Read the model definition and answer for the solid it produces. Units are mm, in the model's axes. Face numbers are marked on the shaded views. A direction names the side the tool comes from. Coordinates: 2 decimals unless noted, no trailing zeros. Write each loop counter-clockwise with the first axis right and the second up, starting at its lowest first coordinate (ties: lowest second). Pieces come first, ordered by that corner, then holes. Notation, with made-up numbers: (61, 71.25) -> (113, 71.25) arc R21 ccw to (113, 89.25) -> close; hole circle Ø1 at (66, 41). An arc over 180 degrees is marked (long way). One line per item, written item: value. Start each with the question number.
from build123d import *

# Parameters (mm, degrees)
SALIENTE_EXTRUIR1_DEPTH = 18
CROQUIS2_R              = 2.5
CORTAR_EXTRUIR1_DEPTH   = 2.5
CROQUIS3_W              = 13
CROQUIS3_H              = 3
CORTAR_EXTRUIR2_DEPTH   = 47.14108798
CHAFL_N1_SIZE           = 1
CHAFL_N2_SIZE           = 1
CHAFL_N2_SIZE2          = 2.087588248
CROQUIS4_W              = 8
CROQUIS4_H              = 12
SALIENTE_EXTRUIR2_DEPTH = 2
CROQUIS5_R              = 1
CORTAR_EXTRUIR3_DEPTH   = 46.169126624
CHAFL_N3_SIZE           = 3
CHAFL_N4_SIZE           = 2


with BuildPart() as part:
    # Croquis1 → Saliente-Extruir1 (new body)
    with BuildSketch(Plane(origin=(0, 0, 0), x_dir=(1, 0, 0), z_dir=(0, 1, 0))):
        Polygon((4, -1.5), (38, -17.5), (38, -14.5), (4, 1.5), (-4, 1.5), (-4, -1.5), align=None)
    extrude(amount=SALIENTE_EXTRUIR1_DEPTH)

    # Croquis2 → Cortar-Extruir1 (cut)
    with BuildSketch(Plane(origin=(0, 0, -1.5), x_dir=(-1, 0, 0), z_dir=(0, 0, -1))):
        with Locations((0, 9)):
            Circle(CROQUIS2_R)
    extrude(amount=-CORTAR_EXTRUIR1_DEPTH, mode=Mode.SUBTRACT)

    # Croquis3 → Cortar-Extruir2 (cut, through all)
    with BuildSketch(Plane(origin=(0, 0, -1.5), x_dir=(-1, 0, 0), z_dir=(0, 0, -1))):
        with Locations((-2.5, 16.5)):
            Rectangle(CROQUIS3_W, CROQUIS3_H)
        with Locations((-2.5, 1.5)):
            Rectangle(CROQUIS3_W, CROQUIS3_H)
    extrude(amount=-CORTAR_EXTRUIR2_DEPTH, mode=Mode.SUBTRACT)

    # Chaflán1
    chafl_n1_edges = [part.edges().sort_by_distance(p)[0] for p in [
        (23.5, 18, 7.676470588),
        (23.5, 0, 7.676470588),
    ]]
    chamfer(chafl_n1_edges, length=CHAFL_N1_SIZE)

    # Chaflán2
    chafl_n2_edges = [part.edges().sort_by_distance(p)[0] for p in [
        (38, 9, 14.5),
    ]]
    chafl_n2_side = [part.faces().sort_by_distance(p)[0] for p in [
        (38, 9, 16.023643901),
    ]]
    chamfer(chafl_n2_edges, length=CHAFL_N2_SIZE, length2=CHAFL_N2_SIZE2, reference=chafl_n2_side[0])

    # Croquis4 → Saliente-Extruir2 (add)
    with BuildSketch(Plane.XY.offset(1.5)):
        with Locations((0, 9)):
            Rectangle(CROQUIS4_W, CROQUIS4_H)
    extrude(amount=SALIENTE_EXTRUIR2_DEPTH)

    # Croquis5 → Cortar-Extruir3 (cut, through all)
    with BuildSketch(Plane(origin=(0, 0, 1), x_dir=(-1, 0, 0), z_dir=(0, 0, -1))):
        with Locations((0, 9)):
            Circle(CROQUIS5_R)
    extrude(amount=-CORTAR_EXTRUIR3_DEPTH, mode=Mode.SUBTRACT)

    # Chaflán3
    chafl_n3_edges = [part.edges().sort_by_distance(p)[0] for p in [
        (-4, 15, 1),
        (-4, 3, 1),
    ]]
    chamfer(chafl_n3_edges, length=CHAFL_N3_SIZE)

    # Chaflán4
    chafl_n4_edges = [part.edges().sort_by_distance(p)[0] for p in [
        (4, 9, 3.5),
    ]]
    chamfer(chafl_n4_edges, length=CHAFL_N4_SIZE - 0.0001)  # a hair under: the kernel refuses the full size


solid = part.part
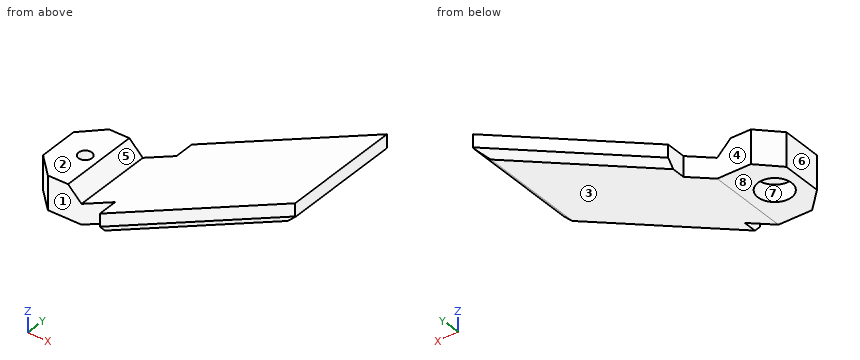
1. Find the intervals of material crossed by probe 1 along Y at (x, z) = (0, -0.35); probe 2 along Y at (x, z) = (0, 2.6); probe 3 along X at (y, z) = (10.5, 12), in increasing order. Write a range as from..to.
2. A cutting plane is placed at D-D on z = 0.25. Give the vertices of the cut face in (x, y).
3. For a pull along X with two mould halves and no side action, classify the marked faces 6, 7 and 8 as +X half, -X half, draft (parallel to the pull), parting line (faces both ways), or undercut.
4. A cutting plane is placed at A-A on x = 0. Give the vertices of the cut face in (y, z).
5. A tool of negligible diameter and unlimited length cuts with its end or side. For the marked faces 1, 2, 3, 4 and 5, from which of +Z, -Z, +X, -X, +Y, -Y can it reach the whole face along a straight path? Write none if from no direction.
6. Given pin 1 (8 mm diameter, centred on x = 20, y = 12, fed in from +Z); pin 2 (1 mm diameter, centred on y = 5, z = 12.5, fed in from -X); pin 3 (5 mm diameter, centred on x = 11.5, y = 2, fed in from +Z); pin 4 (10 mm diameter, centred on x = 27.5, z = 1, fed in from +Y), each flat-ended and moving along its own axis, determine where each tip first touches the part or whether it passes through.
Derived:
1. probe 1: y = 3..6.5, 11.5..15
1. probe 2: y = 3..8, 10..15
1. probe 3: x = 26.31..32.69
2. outline: (-4, 6) -> (-1, 3) -> (7.72, 3) -> (7.72, 15) -> (-1, 15) -> (-4, 12) -> close; hole circle Ø5 at (0, 9)
3. face 6: -X half
3. face 7: undercut
3. face 8: draft
4. outline: (3, -1.5) -> (6.5, -1.5) -> (6.5, 1) -> (8, 1) -> (8, 3.5) -> (3, 3.5) -> close; (10, 1) -> (11.5, 1) -> (11.5, -1.5) -> (15, -1.5) -> (15, 3.5) -> (10, 3.5) -> close
5. face 1: +Z, -Z, -X, -Y
5. face 2: +Z, -X, +Y, -Y
5. face 3: -Z, +X, +Y, -Y
5. face 4: +Z, -Z, -X, +Y
5. face 5: +Z, +Y, -Y
6. pin 1: stops at z = 10.91
6. pin 2: stops at x = 26.31
6. pin 3: stops at z = 6.21
6. pin 4: passes through
